Source: CAD feature listing. Evaluate the final solid. Frame: model axes, mm. Give positions to 0.01 mm unless a question says otherwise; leave off trailing zeros. Loops run counter-clockwise (first coordinate to the right, second up) from the corner with the lowest first, then second, coordinate; pieces in that order, holes last.
```python
from build123d import *

# Parameters (mm, degrees)
CROQUIS1_R              = 27.5
SALIENTE_EXTRUIR1_DEPTH = 20
CORTAR_EXTRUIR1_DEPTH   = 6
VACIADO3_START          = 2
VACIADO3_DEPTH          = 18
VACIADO3_START_2        = 8
VACIADO3_2_DEPTH        = 12


# Read off the part's stored shape, not the designer's step: Vaciado3
with BuildPart() as part:
    # Croquis1 → Saliente-Extruir1 (new body)
    with BuildSketch(Plane(origin=(0, 0, 0), x_dir=(1, 0, 0), z_dir=(0, 1, 0))):
        with Locations(Location((0, 0, 0), (0, 0, 270))):
            Circle(CROQUIS1_R)
    extrude(amount=SALIENTE_EXTRUIR1_DEPTH)

    # Croquis2 → Cortar-Extruir1 (cut)
    with BuildSketch(Plane(origin=(0, 0, 0), x_dir=(-1, 0, 0), z_dir=(0, -1, 0))):
        with BuildLine():
            Line((3.016301233, -22.610051457), (2.862051808, -27.350661042))
            ThreePointArc((2.862051808, -27.350661042), (0.986172274, -27.482311843), (-0.894318642, -27.485454229))
            Line((-0.894318642, -27.485454229), (-0.731715252, -22.488098915))
            Line((-0.731715252, -22.488098915), (3.016301233, -22.610051457))
        make_face()
        with BuildLine():
            Line((0.731715252, 22.488098915), (4.479731738, 22.366146372))
            Line((4.479731738, 22.366146372), (4.633981164, 27.106755958))
            ThreePointArc((4.633981164, 27.106755958), (2.770627687, 27.360073505), (0.894318642, 27.485454229))
            Line((0.894318642, 27.485454229), (0.731715252, 22.488098915))
        make_face()
    extrude(amount=-CORTAR_EXTRUIR1_DEPTH, mode=Mode.SUBTRACT)

    # Vaciado3 outline → Vaciado3 (cut)
    with BuildSketch(Plane(origin=(0, 0, 0), x_dir=(1, 0, 0), z_dir=(0, 1, 0)).offset(VACIADO3_START)):
        with BuildLine():
            ThreePointArc((2.825664836, -25.342959934), (25.486512103, 0.829277286), (1.172219416, 25.473042646))
            Line((1.172219416, 25.473042646), (1.332268229, 20.554198145))
            Line((1.332268229, 20.554198145), (-6.413632508, 20.302162891))
            Line((-6.413632508, 20.302162891), (-6.554878223, 24.643124223))
            ThreePointArc((-6.554878223, 24.643124223), (-25.486512103, -0.829277286), (-4.939039, -25.017112019))
            Line((-4.939039, -25.017112019), (-5.080284715, -20.676150687))
            Line((-5.080284715, -20.676150687), (2.665616022, -20.424115433))
            Line((2.665616022, -20.424115433), (2.825664836, -25.342959934))
        make_face()
    extrude(amount=VACIADO3_DEPTH, mode=Mode.SUBTRACT)

    # Vaciado3 2 outline → Vaciado3 2 (cut)
    with BuildSketch(Plane(origin=(0, 0, 0), x_dir=(1, 0, 0), z_dir=(0, 1, 0)).offset(VACIADO3_START_2)):
        with BuildLine():
            Line((1.332268229, 20.554198145), (1.172219416, 25.473042646))
            ThreePointArc((1.172219416, 25.473042646), (-2.723131489, 25.354182197), (-6.554878223, 24.643124223))
            Line((-6.554878223, 24.643124223), (-6.413632508, 20.302162891))
            Line((-6.413632508, 20.302162891), (1.332268229, 20.554198145))
        make_face()
        with BuildLine():
            ThreePointArc((-4.939039, -25.017112019), (-1.069173421, -25.477575791), (2.825664836, -25.342959934))
            Line((2.825664836, -25.342959934), (2.665616022, -20.424115433))
            Line((2.665616022, -20.424115433), (-5.080284715, -20.676150687))
            Line((-5.080284715, -20.676150687), (-4.939039, -25.017112019))
        make_face()
    extrude(amount=VACIADO3_2_DEPTH, mode=Mode.SUBTRACT)


solid = part.part
```
(1) Section B-B, the plane z = 0. Return the cut outline in (x, y).
A:
outline: (-27.5, 0) - (27.5, 0) - (27.5, 20) - (25.5, 20) - (25.5, 2) - (-25.5, 2) - (-25.5, 20) - (-27.5, 20) - close
(2) Mould query, pull axis Z, two halves, no side actions, for faces 1 (the cylindrical face through (-10.533, 9.86, 25.403)), 2 (the flat face through (-18.2, 20, 18.2)), 3 (the flat face through (0, 2, 0)). Classes: pulls with the +Z half, pulls with the -Z half, needs draft (parallel to the pull), parting line crosses it, or undercut.
A:
face 1: parting line crosses it
face 2: needs draft
face 3: undercut
(3) First-contact query: pin 1 (3 mm diameter, centred on y = 15.5, z = 10.5, fed in from +X); pin 2 (5 mm diameter, centred on x = 1, y = 14.5, fed in from -Z); pin 3 (4 mm diameter, centred on x = -19.5, y = 11.5, fed in from +Z); pin 4 (4 mm diameter, centred on x = -4.5, z = -23, fed in from +Y). Flat tips, straight axial feed; report the tip coordinate or a pass-through.
A:
pin 1: stops at x = 25.99
pin 2: stops at z = -27.5
pin 3: stops at z = 21.21
pin 4: stops at y = 8
(4) Ray query, line 1 along Y through (x, z) = (7.5, -9); line 2 along X through (y, z) = (2.5, 10); line 3 along Z through (x, y) = (-18, 7.5). Return the intervals inside material, ascending.
A:
line 1: y = 0 to 2
line 2: x = -25.62 to -23.46, 23.46 to 25.62
line 3: z = -20.79 to -18.06, 18.06 to 20.79
(5) Section C-C, the plane x = -14.5. Return the cut outline in (y, z), then the cut area to 3 significant figures.
A:
outline: (0, -23.37) - (20, -23.37) - (20, -20.98) - (2, -20.98) - (2, 20.98) - (20, 20.98) - (20, 23.37) - (0, 23.37) - close
area: 180 mm2
(6) Section D-D, the plane x = 0. Return the cut outline in (y, z).
A:
outline: (0, -27.5) - (20, -27.5) - (20, -25.5) - (8, -25.5) - (8, -20.51) - (2, -20.51) - (2, 20.51) - (8, 20.51) - (8, 25.5) - (20, 25.5) - (20, 27.5) - (6, 27.5) - (6, 22.51) - (0, 22.51) - close
(7) Section A-A, the plane y = 13. Return the cut outline in (x, z), then the cut area to 3 significant figures.
A:
outline: circle Ø55 at (0, 0); hole circle Ø51 at (0, 0)
area: 333 mm2
